Source: three-view drawing plus pictorial views. Frame: mm from the lowest corner of the part. Give positions to 0.01 mm unless a question says otherwise; leave off trailing zeros. Write each loop counter-clockwise with the first axis right and the second up, starting at its lowest first coordinate (ties: lowest second). Pieces come first, ordered by that corner, then holes. Notation, with made-up numbers: (-20, 56) -> (33, 56) arc R10 cw to (33, 72) -> close; hole circle Ø5 at (-2, -21.75). An arc over 180 degrees is marked (long way). Answer in a Markdown table with one row per item. Add a question column.
Item 1: Material intervals for probe 1 along Z at (x, y) = (127, 2.25); probe 2 along X at (y, z) = (1.5, 23); probe 3 along X at (y, z) = (5.5, 90) (1 decimal), sorted ascending. Write a range as from..to.
Item 2: First-contact query: P1, Ø3, axis at x = 152.4, z = 88.9, coming from the +Y side. Flat tip, straight axial feed; report the tip coordinate or a pass-through.
Item 3: Section query A-A on z = 88.9. Output: boundary loops of the cut face in (x, y).
Item 4: Section query D-D on z = 20. Output: boundary loops of the cut face in (x, y).
Item 5: Section query B-B on x = 127. Output: boundary loops of the cut face in (y, z), plus the area to 3 significant figures.
Item 6: Section query C-C on y = 2.5. Output: boundary loops of the cut face in (x, z) (1 decimal), plus the area to 3 significant figures.
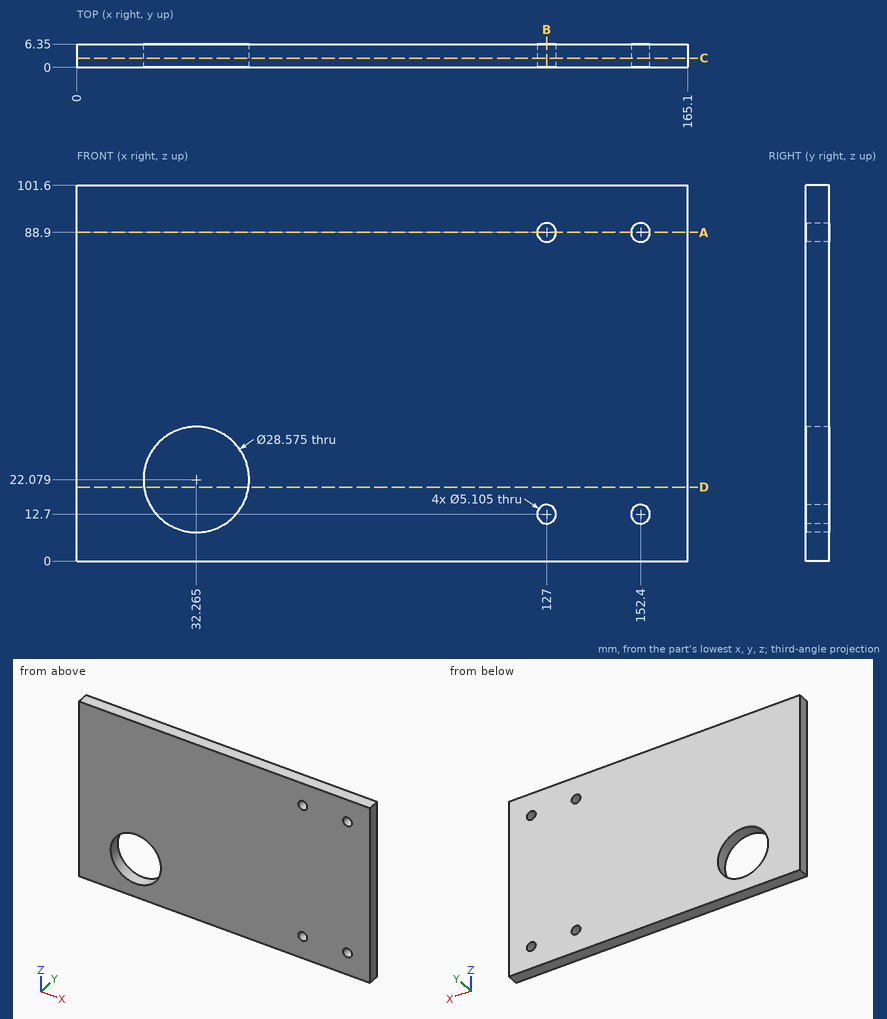
Findings below:
| question | item | result |
|---|---|---|
| 1 | probe 1 | z = 0..10.15, 15.25..86.35, 91.45..101.6 |
| 1 | probe 2 | x = 0..18.01, 46.52..165.1 |
| 1 | probe 3 | x = 0..124.7, 129.3..150.1, 154.7..165.1 |
| 2 | P1 | passes through |
| 3 | outline | (0, 0) -> (124.45, 0) -> (124.45, 6.35) -> (0, 6.35) -> close; (129.55, 0) -> (149.85, 0) -> (149.85, 6.35) -> (129.55, 6.35) -> close; (154.95, 0) -> (165.1, 0) -> (165.1, 6.35) -> (154.95, 6.35) -> close |
| 4 | outline | (0, 0) -> (18.13, 0) -> (18.13, 6.35) -> (0, 6.35) -> close; (46.4, 0) -> (165.1, 0) -> (165.1, 6.35) -> (46.4, 6.35) -> close |
| 5 | outline | (0, 0) -> (6.35, 0) -> (6.35, 10.15) -> (0, 10.15) -> close; (0, 15.25) -> (6.35, 15.25) -> (6.35, 86.35) -> (0, 86.35) -> close; (0, 91.45) -> (6.35, 91.45) -> (6.35, 101.6) -> (0, 101.6) -> close |
| 5 | area | 580 mm^2 |
| 6 | outline | (0, 0) -> (165.1, 0) -> (165.1, 101.6) -> (0, 101.6) -> close; hole circle Ø28.6 at (32.3, 22.1); hole circle Ø5.1 at (127, 12.7); hole circle Ø5.1 at (127, 88.9); hole circle Ø5.1 at (152.4, 12.7); hole circle Ø5.1 at (152.4, 88.9) |
| 6 | area | 16,100 mm^2 |
